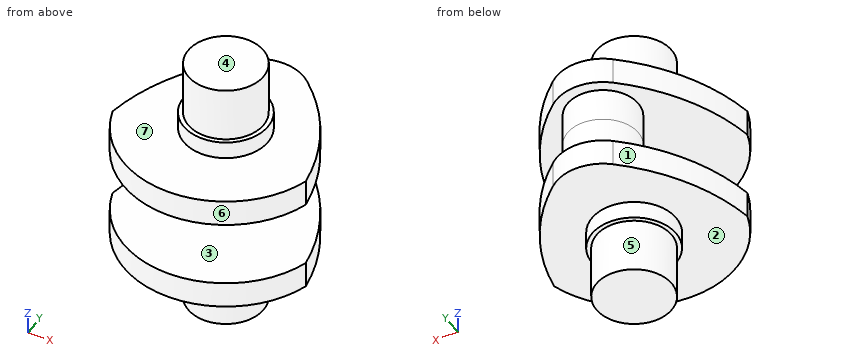
from build123d import *

# Parameters (mm, degrees)
SKETCH1_R           = 170
BOSS_EXTRUDE1_DEPTH = 250
SKETCH2_R           = 190
BOSS_EXTRUDE2_DEPTH = 80
BOSS_EXTRUDE3_DEPTH = 120
SKETCH4_R           = 160
BOSS_EXTRUDE4_DEPTH = 150


with BuildPart() as part:
    # Sketch1 → Boss-Extrude1 (new body)
    with BuildSketch(Plane.XY):
        Circle(SKETCH1_R)
    extrude(amount=BOSS_EXTRUDE1_DEPTH)

    # Sketch2 → Boss-Extrude2 (add)
    with BuildSketch(Plane(origin=(0, 0, 0), x_dir=(-1, 0, 0), z_dir=(0, 0, -1))):
        Circle(SKETCH2_R)
    extrude(amount=BOSS_EXTRUDE2_DEPTH)

    # Sketch3 → Boss-Extrude3 (add)
    with BuildSketch(Plane(origin=(0, 0, -80), x_dir=(-1, 0, 0), z_dir=(0, 0, -1))):
        with BuildLine():
            ThreePointArc((-440, -134.16407865), (0, -460), (440, -134.16407865))
            ThreePointArc((440, -134.16407865), (336.834442487, 164.692576238), (136.680947576, 409.431234611))
            ThreePointArc((136.680947576, 409.431234611), (0, 460), (-136.680947576, 409.431234611))
            ThreePointArc((-136.680947576, 409.431234611), (-336.834442487, 164.692576238), (-440, -134.16407865))
        make_face()
    extrude(amount=BOSS_EXTRUDE3_DEPTH)

    # Sketch4 → Boss-Extrude4 (add)
    with BuildSketch(Plane(origin=(0, 0, -200), x_dir=(-1, 0, 0), z_dir=(0, 0, -1))):
        with Locations((0, 250)):
            Circle(SKETCH4_R)
    extrude(amount=BOSS_EXTRUDE4_DEPTH)

    # Mirror1: part across plane


with BuildPart() as part_1:
    add(part.part)
    add(part.part.mirror(Plane(origin=(0, 250, -350), x_dir=(1, 0, 0), z_dir=(0, 0, -1))))


solid = part_1.part
Can you work these out from the model? Positions are in its coordinate system, mm. Face numbers are marked on the shaded views. A direction names the side the tool comes from. Round coordinates to 2 decimals unless told otherwise and drop trailing zeros. Loops run counter-clockwise (first coordinate to the right, second up) from the corner with the lowest first, then second, coordinate; pieces in that order, holes last. Notation, with made-up numbers: (66, 30.5) - (93, 30.5) arc R13 cw to (93, 45.5) - close; hole circle Ø11 at (5.5, 56.5). An arc over 180 degrees is marked (long way). Answer in a Markdown table with one row per item. Add a question column.
Q1. I want a section at B-B on x = 0. List the corners of the cut face in (y, z) for me, and give its area (3 significant figures).
Q2. Which directions (+Z, -Z, +X, -X, +Y, -Y) give clear straight access to the entire face, cutting with the end or side of a thin tool? Please do the marked faces 5, 6 and 7.
Q3. I need wall thicknesses on L1, parallel to Z at x = 332, y = -11; L2, parallel to X at y = -329.5, z = -140; L3, parallel to Y at x = -25, z = -759. Which ranges of each line are inside material? Lowest first, please.
Q4. We'd pull the mould along Z, two halves only. Please class the marked faces 1, 2, 3 and 4: pulls with the +Z half, pulls with the -Z half, needs draft (parallel to the pull), parting line crosses it, or undercut.
Q5. I want a section at D-D on z = 27. List the corners of the cut face in (x, y) for me, and give its area (3 significant figures).
Q6. I want a section at C-C on y = 250. List the corners of the cut face in (x, z) for me.
Q7. I want a section at A-A on y = 0. List the corners of the cut face in (x, z) for me, and give its area (3 significant figures).
Q8. For pin 1 Ø1 at (x, y) = (197, -315) entering from +Z; pin 2 Ø5 at (x, z) = (52, 125.5) entering from -Y; pin 3 Ø6 at (y, z) = (-125, -102.5) entering from +X, each with a flat end and sliding along its axis, tell me the tip position at first contact or that it passes through.
A:
| question | item | result |
|---|---|---|
| 1 | outline | (-460, -620) - (-190, -620) - (-190, -700) - (-170, -700) - (-170, -950) - (170, -950) - (170, -700) - (190, -700) - (190, -620) - (460, -620) - (460, -500) - (410, -500) - (410, -200) - (460, -200) - (460, -80) - (190, -80) - (190, 0) - (170, 0) - (170, 250) - (-170, 250) - (-170, 0) - (-190, 0) - (-190, -80) - (-460, -80) - (-460, -200) - (90, -200) - (90, -500) - (-460, -500) - close |
| 1 | area | 548,000 mm^2 |
| 2 | face 5 | -Z |
| 2 | face 6 | +Z, -Z, -Y |
| 2 | face 7 | +Z |
| 3 | L1 | -620 to -500, -200 to -80 |
| 3 | L2 | -320.98 to 320.98 |
| 3 | L3 | -168.15 to 168.15 |
| 4 | face 1 | needs draft |
| 4 | face 2 | pulls with the -Z half |
| 4 | face 3 | undercut |
| 4 | face 4 | pulls with the +Z half |
| 5 | outline | circle Ø340 at (0, 0) |
| 5 | area | 90,800 mm^2 |
| 6 | outline | (-282.74, -620) - (282.74, -620) - (282.74, -500) - (160, -500) - (160, -200) - (282.74, -200) - (282.74, -80) - (-282.74, -80) - (-282.74, -200) - (-160, -200) - (-160, -500) - (-282.74, -500) - close |
| 7 | outline | (-408.23, -620) - (-190, -620) - (-190, -700) - (-170, -700) - (-170, -950) - (170, -950) - (170, -700) - (190, -700) - (190, -620) - (408.23, -620) - (408.23, -500) - (-408.23, -500) - close; (-408.23, -200) - (408.23, -200) - (408.23, -80) - (190, -80) - (190, 0) - (170, 0) - (170, 250) - (-170, 250) - (-170, 0) - (-190, 0) - (-190, -80) - (-408.23, -80) - close |
| 7 | area | 427,000 mm^2 |
| 8 | pin 1 | z = -80 |
| 8 | pin 2 | y = -162.63 |
| 8 | pin 3 | x = 439.01 |
